```python
from build123d import *

# Parameters (mm, degrees)
F0_W          = 25
F0_H          = 20
F1_DEPTH      = 10
F4_W          = 2
F4_H          = 5
F4_W_2        = 1
F4_H_2        = 1
F5_DEPTH      = 25
F5_DEPTH_BACK = 25
F6_DEPTH      = 0.5
F7_DEPTH      = 0.5
F8_W          = 4.63
F8_H          = 4.5
F8_W_2        = 6.37
F8_H_2        = 6.5
F9_DEPTH      = 25
F10_W         = 1
F10_H         = 8.375
F11_DEPTH     = 0.5
F12_W         = 3.5
F12_H         = 2.5
F13_DEPTH     = 5
F14_W         = 3
F14_H         = 2
F15_DEPTH     = 5


with BuildPart() as f1:
    # F0 (on Top) → F1 (new body)
    with BuildSketch(Plane.XY):
        with Locations((7.5, 0)):
            Rectangle(F0_W, F0_H)
    extrude(amount=-F1_DEPTH)

    # F2 (on Top) → F3 (revolve, cut)
    with BuildSketch(Plane.XY):
        with BuildLine():
            Line((3.225, 0), (-1.475, 0))
            ThreePointArc((-1.475, 0), (-1.0429825023, -1.0429825023), (0, -1.475))
            Line((0, -1.475), (2.125, -1.475))
            Line((2.125, -1.475), (2.125, -1.625))
            Line((2.125, -1.625), (3.225, -1.625))
            Line((3.225, -1.625), (3.225, 0))
        make_face()
    revolve(axis=Axis((-2.855158034, 0, 0), (-1, 0, 0)), mode=Mode.SUBTRACT)

    # F4 (on Front) → F5 (cut, two sides)
    with BuildSketch(Plane.XZ) as f5_sk:
        with Locations((6.63, -2.5)):
            Rectangle(F4_W, F4_H)
        with Locations((3.63, -0.5)):
            Rectangle(F4_W_2, F4_H_2)
    extrude(amount=-F5_DEPTH, mode=Mode.SUBTRACT)
    extrude(f5_sk.sketch, amount=F5_DEPTH_BACK, mode=Mode.SUBTRACT)

    # F6 (cut): faces of the model
    f6_faces = [f1.faces().sort_by_distance(p)[0] for p in [
        (4.88, 0, 0),
        (13.815, 0, 0),
    ]]
    extrude(f6_faces, amount=-F6_DEPTH, mode=Mode.SUBTRACT)

    # F7 (add): a face of the model
    f7_faces = [f1.faces().sort_by_distance(p)[0] for p in [
        (2.9141072257, 5.8125, 0),
    ]]
    extrude(f7_faces, amount=F7_DEPTH)

    # F8 (on face) → F9 (cut)
    with BuildSketch(Plane.XZ.offset(10)):
        with Locations((0.315, -7.75)):
            Rectangle(F8_W, F8_H)
        with Locations((13.815, -6.75)):
            Rectangle(F8_W_2, F8_H_2)
    extrude(amount=-F9_DEPTH, mode=Mode.SUBTRACT)

    # F10 (on face) → F11 (join)
    with BuildSketch(Plane.XY.offset(-1)):
        with Locations((3.63, -5.8125)):
            Rectangle(F10_W, F10_H)
        with Locations((3.63, 5.8125)):
            Rectangle(F10_W, F10_H)
    extrude(amount=F11_DEPTH)

    # F12 (on face) → F13 (cut)
    with BuildSketch(Plane.XZ.offset(10)):
        with Locations((6.63, -8.75)):
            Rectangle(F12_W, F12_H)
    extrude(amount=-F13_DEPTH, mode=Mode.SUBTRACT)

    # F14 (on face) → F15 (join)
    with BuildSketch(Plane(origin=(0, 10, 0), x_dir=(-1, 0, 0), z_dir=(0, 1, 0))):
        with Locations((-6.63, -9)):
            Rectangle(F14_W, F14_H)
    extrude(amount=F15_DEPTH)


solid = f1.part
```
Geometry check sheet. Reference: the model listing, model coordinates, mm. A direction names the side the tool comes from. Round coordinates to 2 decimals unless told otherwise and drop trailing zeros. Order: outer loops, then holes, each group sorted by start corner. A loop starts at its lowest first (then second) coordinate and runs counter-clockwise, first axis right, second up. Notation, with made-up numbers: (-22, 80) - (-18, 80) arc R34 cw to (-18, 114) - close; hole circle Ø11 at (37, -13). An arc over 180 degrees is marked (long way). Use a Markdown table: item, result. Add a question column.
1) Section check A-A (z = -3). Record the cut outline in (x, y).
2) Section check C-C (y = 2). Record the cut outline in (x, z).
3) Mould release check, pull along X, two halves, no side actions. Record for faces 1 (the flat face through (20, 0, -5)), 2 (the flat face through (5.13, 12, -9)), 3 (the flat face through (4.88, -8, -9)), 4 (the flat face through (7, 3, -10)): released by +X, released by -X, zero draft, split by the parting line, or undercut.
4) Set-up check for faces 5 (the flat face through (7, 0, -5)), 6 (the flat face through (4.4, 0.1, -0.5)), 7 (the flat face through (17, 0, -7)), 8 (the cylindrical face through (2.683, 0.036, -1.625)): record each of +Z, -Z, +X, -X, +Y, -Y from which the full face is reachable in a straight line by a thin tool's end or side.
5) Gauge pin test, flat ends, axial feed: P1, Ø2, axis at y = 13.5, z = -9, coming from the -X side; P2, Ø8, axis at x = 17, y = 8, coming from the +Z side; P3, Ø5, axis at x = 10, z = -5.5, coming from the +Y side. Record the tip position at first contact, or that the pin passes through.
6) Section check B-B (z = -6.5). Record the cut outline in (x, y).
7) Section check D-D (x = 4.5). Record the cut outline in (y, z).
8) Thickness scan on line 1 along X through (y, z) = (4.25, -4.5); line 2 along X through (y, z) = (-5.25, -5.25); line 3 along X through (y, z) = (-4.75, -8.5). Record the ranges inside material, lowest first.
Established:
| question | item | result |
|---|---|---|
| 1 | outline | (-5, -10) - (5.63, -10) - (5.63, 10) - (-5, 10) - close; (7.63, -10) - (20, -10) - (20, 10) - (7.63, 10) - close |
| 2 | outline | (-5, -10) - (-2, -10) - (-2, -5.5) - (2.63, -5.5) - (2.63, -10) - (10.63, -10) - (10.63, -3.5) - (17, -3.5) - (17, -10) - (20, -10) - (20, -0.5) - (7.63, -0.5) - (7.63, -5) - (5.63, -5) - (5.63, -0.5) - (3.13, -0.5) - (3.13, 0.5) - (-5, 0.5) - close |
| 3 | face 1 | released by +X |
| 3 | face 2 | released by -X |
| 3 | face 3 | undercut |
| 3 | face 4 | zero draft |
| 4 | face 5 | +Z, +Y, -Y |
| 4 | face 6 | +Z, +X, +Y, -Y |
| 4 | face 7 | -Z, +Y, -Y |
| 4 | face 8 | +Z |
| 5 | P1 | x = 5.13 |
| 5 | P2 | z = -0.5 |
| 5 | P3 | y = 10 |
| 6 | outline | (-5, -10) - (-2, -10) - (-2, 10) - (-5, 10) - close; (2.63, -10) - (10.63, -10) - (10.63, 10) - (2.63, 10) - close; (17, -10) - (20, -10) - (20, 10) - (17, 10) - close |
| 7 | outline | (-10, -10) - (10, -10) - (10, -0.5) - (-10, -0.5) - close |
| 8 | line 1 | -5 to 5.63, 7.63 to 10.63, 17 to 20 |
| 8 | line 2 | -5 to 10.63, 17 to 20 |
| 8 | line 3 | -5 to -2, 2.63 to 10.63, 17 to 20 |
